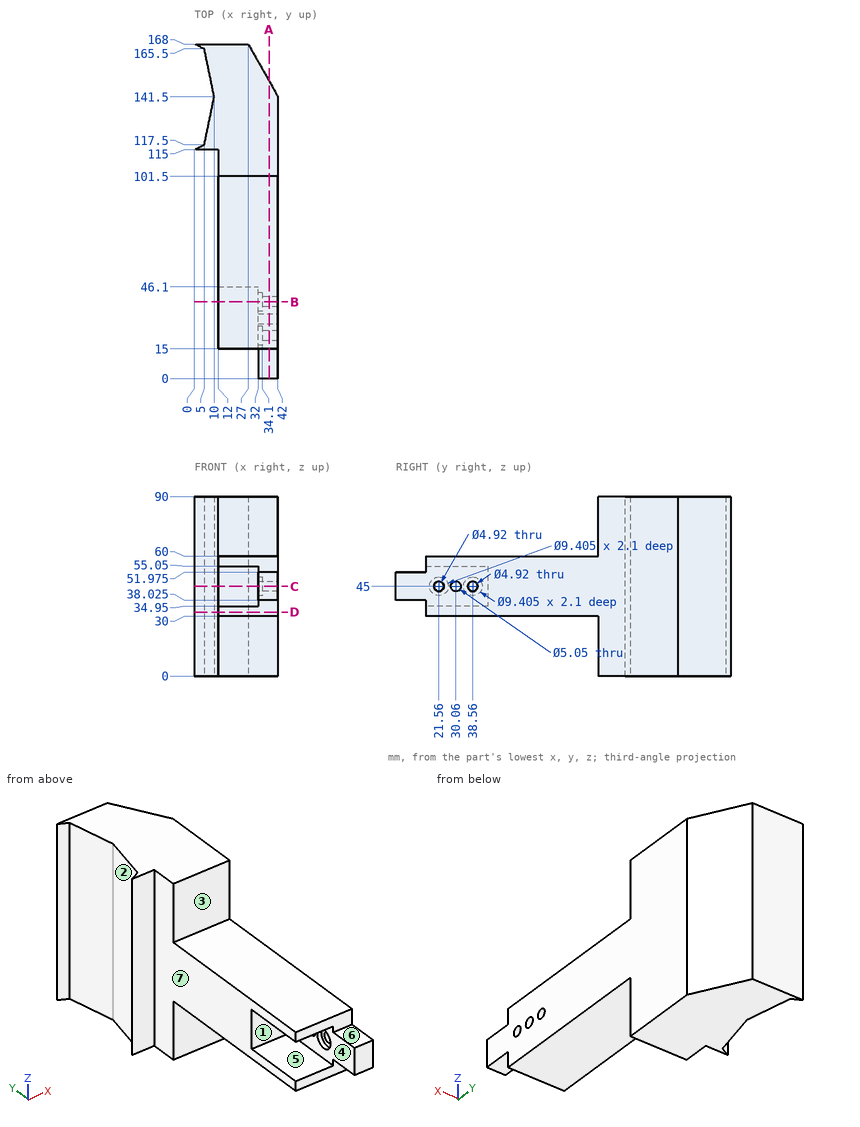
For this review, use the dimensioned drawing (mm, ordinates from the lowest corner) and the shaded views. A direction names the side the tool comes from. Round coordinates to 2 decimals unless told otherwise and drop trailing zeros. Order: outer loops, then holes, each group sorted by start corner. A loop starts at its lowest first (then second) coordinate and runs counter-clockwise, first axis right, second up.
1) Consider section C-C (z = 45). Count the separate pieces of the cut face and the enclosed holes in it, plus the area to 3 significant figures.
The answers:
separate pieces: 4
enclosed holes: 0
area: 4,020 mm2
2) Clearance check with flat-ended pins moving along their axes: pin 1 Ø4 at (x, z) = (29.5, 35) entering from -Y; pin 2 Ø1.5 at (x, y) = (22, 70.5) entering from -Z; pin 3 Ø6 at (y, z) = (82, 25.5) entering from +X; pin 4 Ø2 at (y, z) = (24.5, 45.5) entering from -X. State where each tip first meets the part, or that it passes through.
The answers:
pin 1: stops at y = 15
pin 2: stops at z = 30
pin 3: passes through
pin 4: stops at x = 34.1
3) Machinability: for the marked faces 1, 2 and 3, which of the approach directions +Z, -Z, +X, -X, +Y, -Y give a long, thin tool a straight path to every point of the face, cutting with its end or side? Answer none if there is none.
The answers:
face 1: -X, -Y
face 2: +Z, -Z, -X
face 3: +Z, +X, -X, -Y
4) Consider section D-D (z = 32). State the section outline as (x, y) points, plus the area to 3 significant figures.
The answers:
outline: (0, 115) - (12, 115) - (12, 15) - (42, 15) - (42, 141.5) - (27, 168) - (0, 168) - (5, 165.5) - (10, 141.5) - (5, 117.5) - close
area: 4,650 mm2
5) Draft analysis for pull direction Z (two halves, no side actions). For the marked faces 4, 5, 6 and 7, state which applies: released by +Z, released by -Z, zero draft, split by the parting line, or undercut.
The answers:
face 4: undercut
face 5: undercut
face 6: released by +Z
face 7: zero draft
6) Consider section A-A (x = 37.5). State the section outline as (y, z) points (3 decimals), plus the area to 3 significant figures.
The answers:
outline: (0, 38.025) - (15, 38.025) - (15, 30) - (101.5, 30) - (101.5, 0) - (149.45, 0) - (149.45, 90) - (101.5, 90) - (101.5, 60) - (15, 60) - (15, 51.975) - (0, 51.975) - close; hole circle Ø4.92 at (21.56, 45); hole circle Ø5.05 at (30.06, 45); hole circle Ø4.92 at (38.56, 45)
area: 7,060 mm2
7) For L1, parallel to Z at x = 38, y = 30; L2, parallel to Y at x = 38, z = 45 (3 decimals); L3, parallel to Y at x = 39.25, z = 45 (3 decimals), list the stretches that pass through material, from the lowest coordinate up.
The answers:
L1: z = 30 to 42.48, 47.52 to 60
L2: y = 0 to 19.1, 24.02 to 27.535, 32.585 to 36.1, 41.02 to 148.567
L3: y = 0 to 19.1, 24.02 to 27.535, 32.585 to 36.1, 41.02 to 146.358
8) Consider section B-B (y = 38.56). State the section outline as (x, z) points, plus the area to 3 significant figures.
The answers:
outline: (12, 30) - (42, 30) - (42, 42.54) - (34.1, 42.54) - (34.1, 40.3) - (32, 40.3) - (32, 34.95) - (12, 34.95) - close; (12, 55.05) - (32, 55.05) - (32, 49.7) - (34.1, 49.7) - (34.1, 47.46) - (42, 47.46) - (42, 60) - (12, 60) - close
area: 439 mm2
